Source: CAD feature listing. Evaluate the final solid. Frame: model axes, mm. A direction names the side the tool comes from. Give positions to 0.01 mm unless a question says otherwise; leave off trailing zeros. Write each loop counter-clockwise with the first axis right and the second up, starting at its lowest first coordinate (ties: lowest second). Pieces come first, ordered by that corner, then holes. Notation, with made-up numbers: (54.25, 78.25) - (100.25, 78.25) arc R24 cw to (100.25, 116.25) - close; hole circle Ø5 at (20.5, 0.5). An arc over 180 degrees is marked (long way). One line per question, with ' | ' between items. Start each with the question number.
(1) Pin query (flat end, axial travel): pin 1 (2.5 mm diameter, centred on x = 6.5, y = -22.5, fed in from +Z); pin 2 (0.6 mm diameter, centred on x = -28, z = -4.5, fed in from +Y); pin 3 (3 mm diameter, centred on y = -1, z = 0.5, fed in from +X); pin 4 (12 mm diameter, centred on x = 0, y = 0, fed in from +Z). Return the tip coordinate at first contact, or that it passes through.
(2) Ray query, line 1 (Y direction, x = 0, z = 1.8) (3 decimals); line 2 (Y direction, x = 9, z = -2); line 3 (Y direction, x = -2, z = -2). Return the intervals inside material, ascending. Write a range as [from, to].
(3) Access query for faces 1 (the flat face through (-4.064, 27, -4)), 2 (the flat face through (4, -12, -3.023)), 3 (the flat face through (-6, 22, -0.127)). Directions: +Z, -Z, +X, -X, +Y, -Y. A direction counts if a zero-diameter tool reaches every point of the face in a straight line with its end or side. Return the directions, or none.
(4) Section B-B, the plane z = 1.75. Return loops of the section in (x, y) (3 decimals).
(5) Section D-D, the plane y = 21. Return loops of the section in (x, z), plus the area to 3 significant figures.
(6) Draft query along X for faces 4 (the flat face through (4.064, -27, -4)), 5 (the flat face through (-27, -4.064, -4)), 6 (the flat face through (-5.45, 9.57, 0.79)), 7 (the flat face through (-27.705, 6.396, -0.734)). Return one class per face: +X half, -X half, draft (parallel to the pull), parting line (faces both ways), or undercut.
(7) Section A-A, the plane z = -4. Return loops of the section in (x, y).
```python
from build123d import *

# Parameters (mm, degrees)
SKETCH1_R           = 29.464
BASE_EXTRUDE_DEPTH  = 1.4478
SKETCH2_R           = 18.5674
BOSS_EXTRUDE1_DEPTH = 1.5748
FILLET1_R           = 1.5748
SKETCH3_R           = 17.907
CUT_EXTRUDE1_DEPTH  = 2.032
CUT_EXTRUDE1_DRAFT  = -30
BOSS_EXTRUDE2_DEPTH = 5.715
CUT_EXTRUDE2_START  = -5.715
CUT_EXTRUDE2_DEPTH  = 5.715
SKETCH6_R           = 10.16
CUT_EXTRUDE3_DEPTH  = 43.204498141
CUT_EXTRUDE4_DEPTH  = 42.983088269
CIRPATTERN1_COUNT   = 4
BOSS_EXTRUDE3_DEPTH = 5.9944
CUT_EXTRUDE5_DEPTH  = 4.4704
CIRPATTERN2_COUNT   = 4
CUT_EXTRUDE6_DEPTH  = 0.127
CUT_EXTRUDE7_DEPTH  = 0.127
SKETCH13_RX         = 2.8702
SKETCH13_RY         = 2.315943611
SKETCH13_RX_2       = 1.966975065
SKETCH13_RY_2       = 1.574218937
SKETCH13_RY_3       = 2.01509994
SKETCH13_RX_3       = 1.966974984
SKETCH13_RY_4       = 1.436201162
CUT_EXTRUDE8_DEPTH  = 0.127
CHAMFER1_SIZE       = 1.905


# Read off the part's stored shape, not the designer's step: Cut-Extrude2
with BuildPart() as part:
    # Sketch1 → Base-Extrude (new body)
    with BuildSketch(Plane.XY):
        Circle(SKETCH1_R)
    extrude(amount=-BASE_EXTRUDE_DEPTH)

    # Sketch2 → Boss-Extrude1 (add)
    with BuildSketch(Plane(origin=(0, 0, -1.4478), x_dir=(-1, 0, 0), z_dir=(0, 0, -1))):
        with Locations(Location((0, 0, 0), (0, 0, 180))):
            Circle(SKETCH2_R)
    extrude(amount=BOSS_EXTRUDE1_DEPTH)

    # Fillet1
    fillet1_edges = [part.edges().sort_by_distance(p)[0] for p in [
        (-18.5674, 0, -3.0226),
    ]]
    fillet(fillet1_edges, radius=FILLET1_R - 0.0001)  # a hair under: the kernel refuses the full size


with BuildPart() as cut_extrude1_tool:
    # Sketch3 → Cut-Extrude1 (with draft: the straight prism first)
    with BuildSketch(Plane.XY):
        Circle(SKETCH3_R)
    extrude(amount=-CUT_EXTRUDE1_DEPTH)
    # Cut-Extrude1: the draft: its side faces are tilted about the plane it starts from
    cut_extrude1_sides = [cut_extrude1_tool.faces().sort_by_distance(p)[0] for p in [
        (-17.907, 0, -1.016),
    ]]
    draft(cut_extrude1_sides, Plane.XY, CUT_EXTRUDE1_DRAFT)


with BuildPart() as part_1:
    add(part.part)

    # Cut-Extrude1: cut by cut_extrude1_tool
    add(cut_extrude1_tool.part, mode=Mode.SUBTRACT)

    # Sketch4 → Boss-Extrude2 (add)
    with BuildSketch(Plane.XY.offset(-2.032)):
        Polygon((0, 12.714292158), (-11.0109, 6.357146079), (-11.0109, -6.357146079), (0, -12.714292158), (11.0109, -6.357146079), (11.0109, 6.357146079), align=None)
    extrude(amount=BOSS_EXTRUDE2_DEPTH)

    # Cut-Extrude2 outline → Cut-Extrude2 (cut)
    with BuildSketch(Plane.XY.offset(3.683).offset(CUT_EXTRUDE2_START)):
        with BuildLine():
            ThreePointArc((-11.0109, 4.931967781), (-10.448596497, 6.0325), (-9.776659389, 7.069735228))
            Line((-9.776659389, 7.069735228), (-11.0109, 6.357146079))
            Line((-11.0109, 6.357146079), (-11.0109, 4.931967781))
        make_face()
        with BuildLine():
            Line((0, 12.714292158), (-1.234240611, 12.001703009))
            ThreePointArc((-1.234240611, 12.001703009), (0, 12.065), (1.234240611, 12.001703009))
            Line((1.234240611, 12.001703009), (0, 12.714292158))
        make_face()
        with BuildLine():
            ThreePointArc((-9.776659389, -7.069735228), (-10.448596497, -6.0325), (-11.0109, -4.931967781))
            Line((-11.0109, -4.931967781), (-11.0109, -6.357146079))
            Line((-11.0109, -6.357146079), (-9.776659389, -7.069735228))
        make_face()
        with BuildLine():
            Line((11.0109, 6.357146079), (9.776659389, 7.069735228))
            ThreePointArc((9.776659389, 7.069735228), (10.448596497, 6.0325), (11.0109, 4.931967781))
            Line((11.0109, 4.931967781), (11.0109, 6.357146079))
        make_face()
        with BuildLine():
            ThreePointArc((1.234240611, -12.001703009), (0, -12.065), (-1.234240611, -12.001703009))
            Line((-1.234240611, -12.001703009), (0, -12.714292158))
            Line((0, -12.714292158), (1.234240611, -12.001703009))
        make_face()
        with BuildLine():
            Line((11.0109, -6.357146079), (11.0109, -4.931967781))
            ThreePointArc((11.0109, -4.931967781), (10.448596497, -6.0325), (9.776659389, -7.069735228))
            Line((9.776659389, -7.069735228), (11.0109, -6.357146079))
        make_face()
    extrude(amount=CUT_EXTRUDE2_DEPTH, mode=Mode.SUBTRACT)

    # Sketch6 → Cut-Extrude3 (cut, through all)
    with BuildSketch(Plane.XY.offset(3.683)):
        Circle(SKETCH6_R)
    extrude(amount=-CUT_EXTRUDE3_DEPTH, mode=Mode.SUBTRACT)

    # Sketch8 → Cut-Extrude4 (cut, through all)
    with BuildSketch(Plane(origin=(0, 0, -1.4478), x_dir=(-1, 0, 0), z_dir=(0, 0, -1))):
        with BuildLine():
            Line((2.54, 29.354313073), (2.54, 27.314154279))
            ThreePointArc((2.54, 27.314154279), (-1.838860007, 27.370298096), (-6.170857323, 26.728919617))
            Line((-6.170857323, 26.728919617), (-6.627957865, 28.708839589))
            ThreePointArc((-6.627957865, 28.708839589), (-2.069301544, 29.391245076), (2.54, 29.354313073))
        make_face()
    cut_extrude4 = extrude(amount=-CUT_EXTRUDE4_DEPTH, mode=Mode.SUBTRACT)

    # CirPattern1: Cut-Extrude4 ×4 about axis
    cirpattern1_axis = Axis((0, 0, 0), (0, 0, 1))
    for i in range(1, CIRPATTERN1_COUNT):
        add(cut_extrude4.rotate(cirpattern1_axis, i * 360 / CIRPATTERN1_COUNT), mode=Mode.SUBTRACT)

    # Sketch9 → Boss-Extrude3 (add)
    with BuildSketch(Plane(origin=(0, 0, -1.4478), x_dir=(-1, 0, 0), z_dir=(0, 0, -1))):
        with BuildLine():
            Line((4.064, 25.587269647), (4.064, 29.182378244))
            ThreePointArc((4.064, 29.182378244), (-0.541715145, 29.459019683), (-5.134145774, 29.013235655))
            Line((-5.134145774, 29.013235655), (-4.333000099, 25.543092494))
            ThreePointArc((-4.333000099, 25.543092494), (-0.136301756, 25.907641456), (4.064, 25.587269647))
        make_face()
    boss_extrude3 = extrude(amount=BOSS_EXTRUDE3_DEPTH)

    # Sketch10 → Cut-Extrude5 (cut)
    with BuildSketch(Plane.XY.offset(-1.4478)):
        with BuildLine():
            Line((5.134145774, 29.013235655), (4.676387057, 27.030464815))
            ThreePointArc((4.676387057, 27.030464815), (1.07757011, 27.410827544), (-2.54, 27.314154279))
            Line((-2.54, 27.314154279), (-2.54, 29.354313073))
            ThreePointArc((-2.54, 29.354313073), (1.308236036, 29.434942067), (5.134145774, 29.013235655))
        make_face()
    cut_extrude5 = extrude(amount=-CUT_EXTRUDE5_DEPTH, mode=Mode.SUBTRACT)

    # CirPattern2: Boss-Extrude3, Cut-Extrude5 ×4 about axis
    cirpattern2_axis = Axis((0, 0, 0), (0, 0, 1))
    add([boss_extrude3.rotate(cirpattern2_axis, i * 360 / CIRPATTERN2_COUNT) for i in range(1, CIRPATTERN2_COUNT)])
    add([cut_extrude5.rotate(cirpattern2_axis, i * 360 / CIRPATTERN2_COUNT) for i in range(1, CIRPATTERN2_COUNT)], mode=Mode.SUBTRACT)

    # Sketch11 → Cut-Extrude6 (cut)
    with BuildSketch(Plane.XY):
        Polygon((-7.366154253, 24.742996139), (-5.880429407, 19.198195525), (-4.506496511, 19.566339735), (-5.992221358, 25.111140348), align=None)
    extrude(amount=-CUT_EXTRUDE6_DEPTH, mode=Mode.SUBTRACT)

    # Sketch12 → Cut-Extrude7 (cut)
    with BuildSketch(Plane.XY):
        Polygon((2.979852971, -22.210563913), (8.524653584, -20.724839066), (8.892797794, -22.098771961), (3.347997181, -23.584496808), align=None)
    extrude(amount=-CUT_EXTRUDE7_DEPTH, mode=Mode.SUBTRACT)

    # Sketch13 → Cut-Extrude8 (cut)
    # profile 1 of 2: a face of its own
    with BuildSketch(Plane.XY):
        with Locations(Location((23.11032284, 6.450896771), (0, 0, -165))):
            Ellipse(SKETCH13_RX, SKETCH13_RY)
        with Locations(Location((23.11032284, 6.450896771), (0, 0, -165))):
            Ellipse(SKETCH13_RX_2, SKETCH13_RY_2, mode=Mode.SUBTRACT)
    # profile 2 of 2: a face of its own
    with BuildSketch(Plane.XY):
        with Locations(Location((-21.554852577, -5.517100911), (0, 0, -75))):
            Ellipse(SKETCH13_RX, SKETCH13_RY_3)
        with Locations(Location((-21.554852577, -5.517100911), (0, 0, -75))):
            Ellipse(SKETCH13_RX_3, SKETCH13_RY_4, mode=Mode.SUBTRACT)
    extrude(amount=-CUT_EXTRUDE8_DEPTH, mode=Mode.SUBTRACT)

    # Chamfer1
    chamfer1_edges = [part_1.edges().sort_by_distance(p)[0] for p in [
        (-10.16, 0, -3.0226),
    ]]
    chamfer(chamfer1_edges, length=CHAMFER1_SIZE)


solid = part_1.part
```
Check sheet entries:
1) pin 1: z = 0 | pin 2: y = -2.54 | pin 3: x = 27.43 | pin 4: through
2) line 1: [-12.065, -10.16], [10.16, 12.065] | line 2: [-16.13, -14.13], [-7.52, -6.4], [6.4, 7.52], [14.13, 16.13] | line 3: [-27.36, -25.83], [-18.36, -16.63], [-11.56, -10.86], [10.86, 11.56], [16.63, 18.36], [25.83, 27.36]
3) face 1: -Z, -X, +Y | face 2: -Z | face 3: +Z
4) outline: (-11.011, -4.932) arc R12.065 ccw to (-9.777, -7.07) - (-1.234, -12.002) arc R12.065 ccw to (1.234, -12.002) - (9.777, -7.07) arc R12.065 ccw to (11.011, -4.932) - (11.011, 4.932) arc R12.065 ccw to (9.777, 7.07) - (1.234, 12.002) arc R12.065 ccw to (-1.234, 12.002) - (-9.777, 7.07) arc R12.065 ccw to (-11.011, 4.932) - close; hole circle Ø20.32 at (0, 0)
5) outline: (-20.67, -1.45) - (20.67, -1.45) - (20.67, 0) - (-4.89, 0) - (-4.89, -0.13) - (-6.36, -0.13) - (-6.36, 0) - (-20.67, 0) - close | area: 59.7 mm²
6) face 4: +X half | face 5: draft | face 6: undercut | face 7: -X half
7) outline: (-29.35, -2.54) arc R29.46 ccw to (-29.18, -4.06) - (-25.59, -4.06) arc R25.91 cw to (-25.54, 4.33) - (-27.03, 4.68) arc R27.43 ccw to (-27.31, -2.54) - close; (-4.68, -27.03) arc R27.43 ccw to (2.54, -27.31) - (2.54, -29.35) arc R29.46 ccw to (4.06, -29.18) - (4.06, -25.59) arc R25.91 cw to (-4.33, -25.54) - close; (-4.06, 25.59) arc R25.91 cw to (4.33, 25.54) - (4.68, 27.03) arc R27.43 ccw to (-2.54, 27.31) - (-2.54, 29.35) arc R29.46 ccw to (-4.06, 29.18) - close; (25.54, -4.33) - (27.03, -4.68) arc R27.43 ccw to (27.31, 2.54) - (29.35, 2.54) arc R29.46 ccw to (29.18, 4.06) - (25.59, 4.06) arc R25.91 cw to start
